Source: three-view drawing plus pictorial views. Frame: mm from the lowest corner of the part. A direction names the side the tool comes from. Give positions to 0.01 mm unless a question says otherwise; leave off trailing zeros. Loops run counter-clockwise (first coordinate to the right, second up) from the corner with the lowest first, then second, coordinate; pieces in that order, holes last.
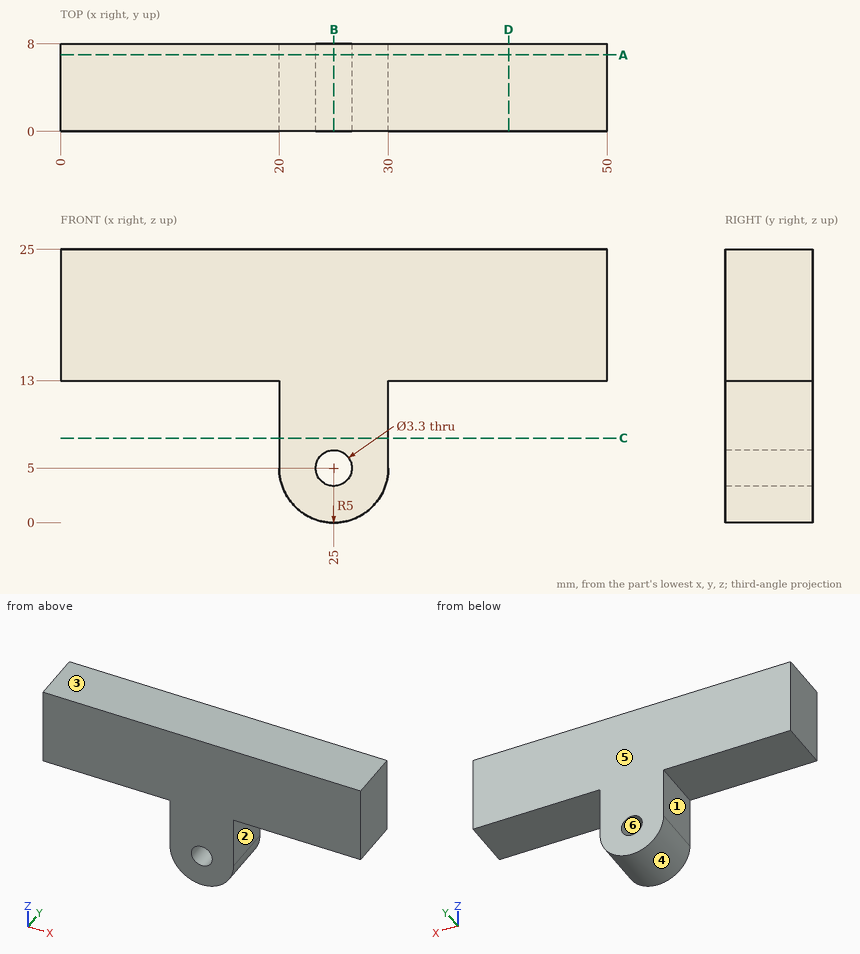
(1) Cut plane D-D (x = 41). Return the cut outline in (y, z), and give its area (3 significant figures).
Values follow:
outline: (0, 13) - (8, 13) - (8, 25) - (0, 25) - close
area: 96.0 mm2
(2) Reachability of the marked faces 1, 2 and 3 from +Z, -Z, +X, -X, +Y, -Y: full face, straight path, thin tool, end or side. Return the list, or none.
Values follow:
face 1: -Z, -X, +Y, -Y
face 2: -Z, +X, +Y, -Y
face 3: +Z, +X, -X, +Y, -Y
(3) Cut plane A-A (y = 7). Return the cut outline in (x, z).
Values follow:
outline: (0, 13) - (20, 13) - (20, 5) arc R5 ccw to (30, 5) - (30, 13) - (50, 13) - (50, 25) - (0, 25) - close; hole circle Ø3.3 at (25, 5)
(4) Cut plane C-C (z = 7.75). Return the cut outline in (x, y), and give its area (3 significant figures).
Values follow:
outline: (20, 0) - (30, 0) - (30, 8) - (20, 8) - close
area: 80.0 mm2
(5) Pin query (flat end, axial travel): pin 1 Ø1 at (y, z) = (2.5, 9) entering from -X; pin 2 Ø2.5 at (y, z) = (5, 8.5) entering from +X; pin 3 Ø2 at (x, y) = (37.5, 2.5) entering from -Z. Return the tip coordinate at first contact, or that it passes through.
Values follow:
pin 1: stops at x = 20
pin 2: stops at x = 30
pin 3: stops at z = 13
(6) Ray query, probe 1 along Z at (x, y) = (25, 4.75); probe 2 along Z at (x, y) = (38.5, 2); probe 3 along X at (y, z) = (7.5, 8). Return the intervals inside material, ascending.
Values follow:
probe 1: z = 0 to 3.35, 6.65 to 25
probe 2: z = 13 to 25
probe 3: x = 20 to 30
(7) Cut plane B-B (x = 25). Return the cut outline in (y, z), and give its area (3 significant figures).
Values follow:
outline: (0, 0) - (8, 0) - (8, 3.35) - (0, 3.35) - close; (0, 6.65) - (8, 6.65) - (8, 25) - (0, 25) - close
area: 174 mm2
(8) Mould query, pull axis X, two halves, no side actions, for the marked faces 4, 5 and 6. Classes: +X half, -X half, draft (parallel to the pull), parting line (faces both ways), or undercut.
Values follow:
face 4: parting line
face 5: draft
face 6: undercut
